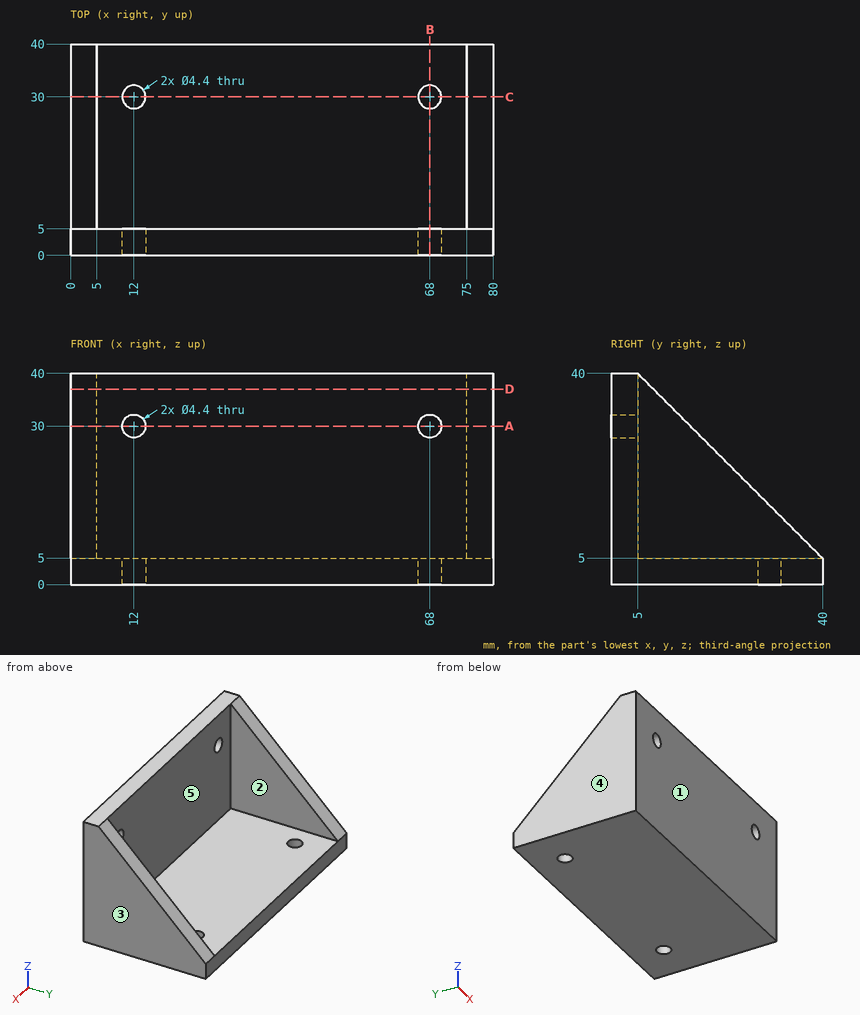
The figure shows three views and two pictorial views of one solid part (mm, origin at its lowest corner). Answer the questions. A direction names the side the tool comes from. Coordinates: 2 decimals unless noted, no trailing zeros. Loops run counter-clockwise (first coordinate to the right, second up) from the corner with the lowest first, then second, coordinate; pieces in that order, holes last.
(1) The part is cut by section D-D (z = 37). Determine the outline of the cut face in (x, y), and give its area (3 significant figures).
Solution:
outline: (0, 0) - (80, 0) - (80, 8) - (75, 8) - (75, 5) - (5, 5) - (5, 8) - (0, 8) - close
area: 430 mm2
(2) The part is cut by section A-A (z = 30). Determine the outline of the cut face in (x, y), and give its area (3 significant figures).
Solution:
outline: (0, 0) - (9.8, 0) - (9.8, 5) - (5, 5) - (5, 15) - (0, 15) - close; (14.2, 0) - (65.8, 0) - (65.8, 5) - (14.2, 5) - close; (70.2, 0) - (80, 0) - (80, 15) - (75, 15) - (75, 5) - (70.2, 5) - close
area: 456 mm2
(3) Consider line 1 along X through (y, z) = (3, 30); line 2 along Y through (x, z) = (68, 2); line 3 along X through (y, z) = (26, 8). Determine where each line is inside the solid, lowest interval first.
Solution:
line 1: x = 0 to 9.8, 14.2 to 65.8, 70.2 to 80
line 2: y = 0 to 27.8, 32.2 to 40
line 3: x = 0 to 5, 75 to 80
(4) Flat-ended cylindrical pins translate along their axes: pin 1 Ø17.5 at (x, z) = (30, 22) entering from +Y; pin 2 Ø4 at (x, z) = (12, 30) entering from -Y; pin 3 Ø6 at (x, y) = (40, 19) entering from +Z. Find the tip coordinate at first contact, or state that the pin passes through.
Solution:
pin 1: stops at y = 5
pin 2: passes through
pin 3: stops at z = 5
(5) A tool of negligible diameter and unlimited length cuts with its end or side. For the marked faces 4 and 5, from which of +Z, -Z, +X, -X, +Y, -Y can it reach the whole face along a straight path? Write none if from no direction.
Solution:
face 4: +Z, -Z, -X, +Y, -Y
face 5: +Z, +Y
(6) The part is cut by section B-B (x = 68). Determine the outline of the cut face in (y, z).
Solution:
outline: (0, 0) - (27.8, 0) - (27.8, 5) - (5, 5) - (5, 27.8) - (0, 27.8) - close; (0, 32.2) - (5, 32.2) - (5, 40) - (0, 40) - close; (32.2, 0) - (40, 0) - (40, 5) - (32.2, 5) - close
(7) The mould has two halves that part along X. Classify the marked faces 1, 2 and 3: released by +X, released by -X, zero draft, split by the parting line, or undercut.
Solution:
face 1: zero draft
face 2: undercut
face 3: released by +X
